Autodesk Inventor part; units mm, degrees
ref_plane "YZ Plane" through (0, 0, 0) normal (1, 0, 0) x (0, 1, 0)
ref_plane "XZ Plane" through (0, 0, 0) normal (0, 1, 0) x (-1, 0, 0)
ref_plane "XY Plane" through (0, 0, 0) normal (0, 0, 1) x (1, 0, 0)
sketch "スケッチ1" plane through (0, 0, 0) normal (0, 0, 1) x (1, 0, 0)
  line L0 (92.493, 12) -> (30.0122, 12)
  arc A0 (30.0122, 12) -> (23.3428, 9.9759) centre (30.0122, 0) ccw
  arc A1 (6.6694, 9.9759) -> (23.3428, 9.9759) centre (15.0061, 22.4459) ccw
  arc A2 (6.6694, 9.9759) -> (0, -12) centre (0, 0) ccw
  line L1 (0, -12) -> (30, -12)
  arc A3 (30, -12) -> (30, -12) centre (30, 0) ccw construction
  line L2 (30, -12) -> (92.493, -12)
  line L3 (92.493, -12) -> (92.493, 12)
  circle A4 centre (30, 0) radius 9.025 construction
  circle A5 centre (0, 0) radius 1.5
  circle A6 centre (16, 0) radius 1.25
  circle A7 centre (48, -5) radius 3.025
  circle A8 centre (73, -5) radius 3.025
  circle A9 centre (60.5, 5) radius 3.025
  line L4 (48, -5) -> (73, -5) construction
  line L5 (92.493, 12) -> (30.0122, 12)
  line L6 (59.7539, 12) -> (92.493, -14.1913)
  line L7 (92.493, -12) -> (92.493, 12)
  line L8 (60.5, 5) -> (73, -5) construction
  line L9 (60.5, 5) -> (60.5, -5) construction
  line L10 (61.2461, 12) -> (28.507, -14.1913)
  arc A10 (44.8765, -1.0957) -> (48, -10) centre (48, -5) ccw
  arc A11 (73, -10) -> (76.1235, -1.0957) centre (73, -5) ccw
  line L11 (48, -10) -> (73, -10)
  point P0 (60.5, 0)
  point P1 (61.3547, 12)
  point P2 (91.3547, -12)
  point P3 (59.6453, 12)
  point P4 (29.6453, -12)
  point P5 (89.7539, -12)
  point P6 (60.5, 11.4031)
  point P7 (31.2461, -12)
  dimension "d0" = 6.05
  dimension "d1" = 6.05
  dimension "d2" = 6.05
  dimension "d3" = 25
  dimension "d4" = 10
  dimension "d5" = 18
  dimension "d6" = 5
extrude "押し出し1" add sketch "スケッチ1" along normal blind 4 contours L6 A11 L11 A10 L10
fillet "フィレット3" radius 6 1 edges at (60.5, 11.4031, 2)
properties part number "アーム詰め物" material "ポリカーボネート、クリア"
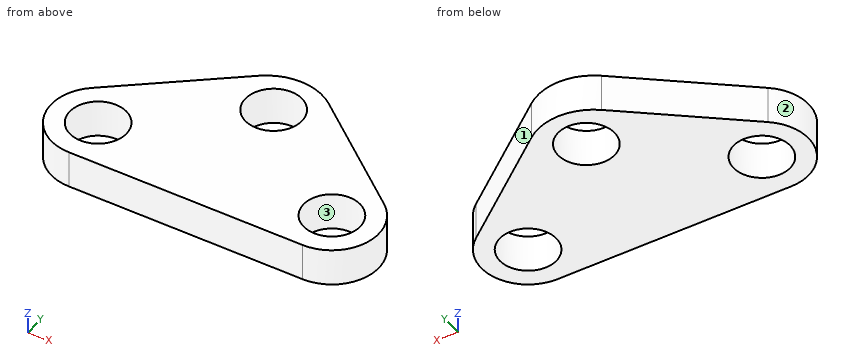
Check sheet for the modelled part. Datum: model origin and axes. Units: mm. Face numbers are marked on the shaded views. Give positions to 0.01 mm unless a question says otherwise; leave off trailing zeros. Loops run counter-clockwise (first coordinate to the right, second up) from the corner with the lowest first, then second, coordinate; pieces in that order, holes last. Notation, with made-up numbers: M 17,-20 L 61,-20 A25 ccw 61,19 Z; hole C 0.25,-35.5 d4. An arc over 180 degrees is marked long. Use a Markdown table: item, result. Add a question column.
Q1. Sectioned sample at B-B, the plane z = 3.3. Give the number of separate pieces and of enclosed holes in the cut face, then the cut area to 3 significant figures.
Q2. Sectioned sample at C-C, the plane x = 60.5. Record the cut outline in (y, z) (3 decimals), then the cut area to 3 significant figures.
Q3. Go/stop test with flat-tipped pins: pin 1 (5 mm diameter, centred on x = 48, y = -5, fed in from +Z); pin 2 (1.5 mm diameter, centred on y = -0.5, z = 1.5, fed in from -X); pin 3 (2 mm diameter, centred on y = -1, z = 0.5, fed in from +X); pin 4 (1.5 mm diameter, centred on x = 64, z = 1, fed in from +Y). Record where each tip stops, or that it passes through.
Q4. Sectioned sample at A-A, the plane y = -5. Record the cut outline in (x, z) (3 decimals).
Q5. Scan lines: line 1 along Y through (x, z) = (60.5, 2) (3 decimals); line 2 along X through (y, z) = (-5.75, 3.4); line 3 along Y through (x, z) = (73, 2.2) (3 decimals). Record each from-to range of solid material in increasing order. Write a range as [from, to].
Q6. Mould release check, pull along Y, two halves, no side actions. Record for the marked faces 1, 2 and 3: pulls with the +Y half, pulls with the -Y half, needs draft (parallel to the pull), parting line crosses it, or undercut.
Q7. Sectioned sample at D-D, the plane y = 5. Record the cut outline in (x, z) (3 decimals), then the cut area to 3 significant figures.
Verdict:
| question | item | result |
|---|---|---|
| 1 | separate pieces | 1 |
| 1 | enclosed holes | 3 |
| 1 | area | 401 mm^2 |
| 2 | outline | M -10,0 L 1.975,0 L 1.975,4 L -10,4 Z; M 8.025,0 L 9.719,0 L 9.719,4 L 8.025,4 Z |
| 2 | area | 54.7 mm^2 |
| 3 | pin 1 | through |
| 3 | pin 2 | x = 44.69 |
| 3 | pin 3 | x = 77 |
| 3 | pin 4 | y = 9.05 |
| 4 | outline | M 43,0 L 44.975,0 L 44.975,4 L 43,4 Z; M 51.025,0 L 69.975,0 L 69.975,4 L 51.025,4 Z; M 76.025,0 L 78,0 L 78,4 L 76.025,4 Z |
| 5 | line 1 | [-10, 1.975], [8.025, 9.719] |
| 5 | line 2 | [43.06, 45.07], [50.93, 70.07], [75.93, 77.94] |
| 5 | line 3 | [-10, -8.025], [-1.975, 1.403] |
| 6 | face 1 | pulls with the +Y half |
| 6 | face 2 | parting line crosses it |
| 6 | face 3 | undercut |
| 7 | outline | M 52.496,0 L 57.475,0 L 57.475,4 L 52.496,4 Z; M 63.525,0 L 68.504,0 L 68.504,4 L 63.525,4 Z |
| 7 | area | 39.8 mm^2 |
